Job drawing, mm, ordinate dimensions from the low corner. One solid piece. A direction names the side the tool comes from. Round coordinates to 2 decimals unless told otherwise and drop trailing zeros. Loops run counter-clockwise (first coordinate to the right, second up) from the corner with the lowest first, then second, coordinate; pieces in that order, holes last.
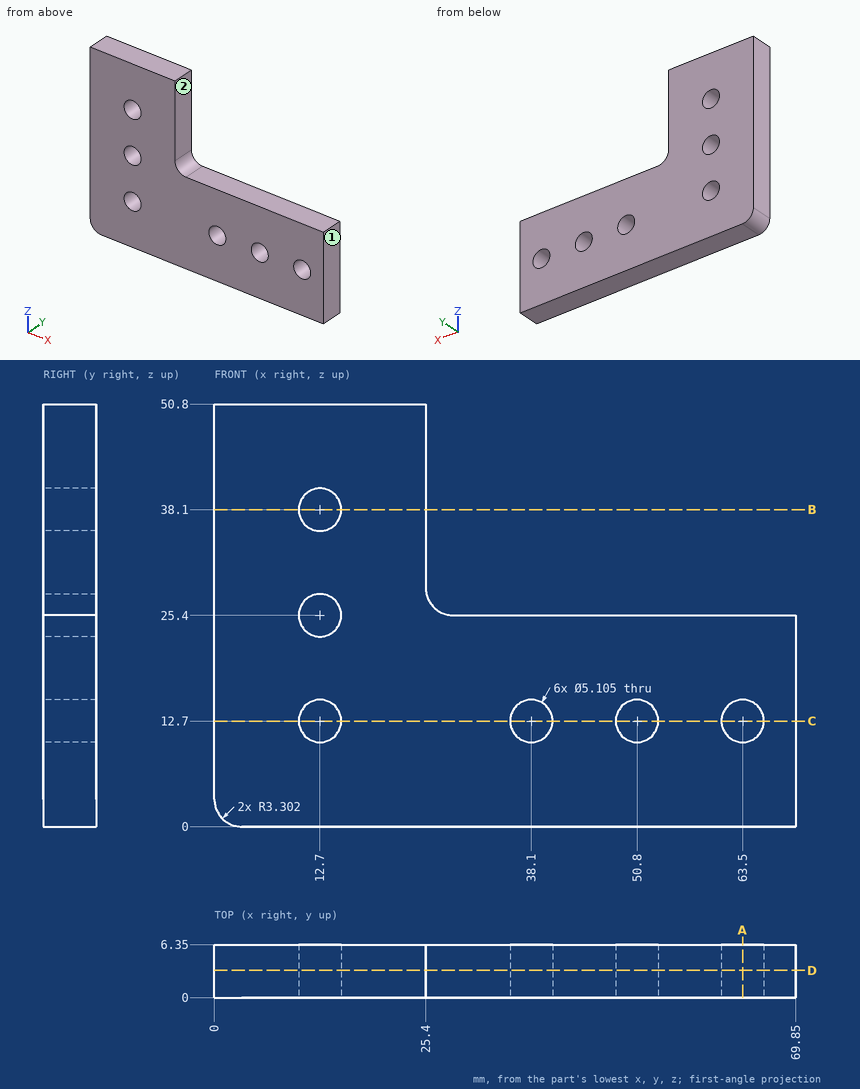
1) Slice it at D-D, the plane y = 3.25. Give the number of separate pieces and of enclosed holes in the cut face, then the cut area to 3 significant figures.
Values:
separate pieces: 1
enclosed holes: 6
area: 2,300 mm2
2) Tool access for the marked faces 1 and 2: list every direction of +Z, -Z, +X, -X, +Y, -Y with a clear straight run to the whole face (end or side of a thin tool).
Values:
face 1: +Z, -Z, +X, +Y, -Y
face 2: +Z, +X, +Y, -Y
3) Wall check: line 1 along X through (y, z) = (2, 12.7); line 2 along Z through (x, y) = (12.7, 4); line 3 along Z through (x, y) = (50.8, 2.25). Give the ranges that are in metal, low to high.
Values:
line 1: x = 0 to 10.15, 15.25 to 35.55, 40.65 to 48.25, 53.35 to 60.95, 66.05 to 69.85
line 2: z = 0 to 10.15, 15.25 to 22.85, 27.95 to 35.55, 40.65 to 50.8
line 3: z = 0 to 10.15, 15.25 to 25.4
4) Slice it at B-B, the plane z = 38.1. Give the cut face in (x, y).
Values:
outline: (0, 0) - (10.15, 0) - (10.15, 6.35) - (0, 6.35) - close; (15.25, 0) - (25.4, 0) - (25.4, 6.35) - (15.25, 6.35) - close
5) Slice it at A-A, the plane x = 63.5. Give the cut face in (y, z).
Values:
outline: (0, 0) - (6.35, 0) - (6.35, 10.15) - (0, 10.15) - close; (0, 15.25) - (6.35, 15.25) - (6.35, 25.4) - (0, 25.4) - close
6) Drop a flat-ended pin along its axis: pin 1 Ø3 at (y, z) = (2, 45) entering from +X. Give the stop position or say it passes through.
Values:
pin 1: stops at x = 25.4
7) Slice it at C-C, the plane z = 12.7. Give the cut face in (x, y), then the cut area to 3 significant figures.
Values:
outline: (0, 0) - (10.15, 0) - (10.15, 6.35) - (0, 6.35) - close; (15.25, 0) - (35.55, 0) - (35.55, 6.35) - (15.25, 6.35) - close; (40.65, 0) - (48.25, 0) - (48.25, 6.35) - (40.65, 6.35) - close; (53.35, 0) - (60.95, 0) - (60.95, 6.35) - (53.35, 6.35) - close; (66.05, 0) - (69.85, 0) - (69.85, 6.35) - (66.05, 6.35) - close
area: 314 mm2
